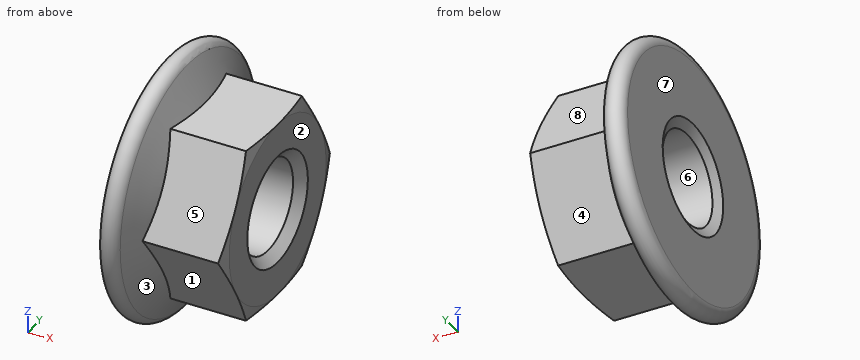
Autodesk Inventor part; units mm, degrees
ref_plane "Work Plane1" through (17.4207, 0, 0) normal (0, 0, -1) x (-1, 0, 0)
ref_plane "YZ Plane" through (0, 0, 0) normal (1, 0, 0) x (0, 1, 0)
ref_plane "XZ Plane" through (0, 0, 0) normal (0, 1, 0) x (-1, 0, 0)
sketch "Sketch1" plane through (0, 0, 0) normal (0, 0, 1) x (1, 0, 0)
  line L0 (-1.1018, 0) -> (6.017, 0)
  line L1 (1.7045, 4) -> (0.9532, 5.6113)
  line L2 (1.7045, 4) -> (5, 4) construction
  line L3 (5, 4) -> (5, 0) construction
  arc A0 (0.9532, 5.6113) -> (0, 5.4) centre (0.5, 5.4) ccw
  line L4 (1.7045, 4) -> (1.7045, 0)
  line L5 (0, -1.1988) -> (0, 7.1926)
  point P0 (0, 0)
  dimension "d2" = 8
  dimension "d4" = 11.8
  dimension "d5" = 0.5
  dimension "d15" = 5
  dimension "d16" = 25
revolve "Ring" add sketch "Sketch1" angle 360 about axis through (-10, 0, 0) along (1, 0, 0)
sketch "Sketch2" plane through (0, 0, 0) normal (-1, 0, 0) x (0, 0, 1)
  circle A0 centre (0, 0) radius 4.9
  line L0 (-4, -2.3094) -> (-4, 2.3094)
  line L1 (-4, 2.3094) -> (0, 4.6188)
  line L2 (0, 4.6188) -> (4, 2.3094)
  line L3 (4, 2.3094) -> (4, -2.3094)
  line L4 (4, -2.3094) -> (0, -4.6188)
  line L5 (0, -4.6188) -> (-4, -2.3094)
  circle A1 centre (0, 0) radius 5.4
  dimension "d6" = 9.2376
extrude "Body" add sketch "Sketch2" against normal blind 5 contours L0 L1 L2 L3 L4 L5
sketch "Sketch3" plane through (0, 0, 0) normal (0, 0, 1) x (1, 0, 0)
  line L0 (1.416, 4.6188) -> (5, 4.6188)
  line L1 (5, 2.3094) -> (5, 4.6188)
  line L2 (0, -5.4) -> (0, 5.4)
  line L3 (-1, 0) -> (6, 0)
  line L4 (4.8342, 4.6188) -> (5, 4)
  dimension "d10" = 15
  dimension "d11" = 8
revolve "Chamfer1" cut sketch "Sketch3" angle 360 about axis through (-10, 0, 0) along (1, 0, 0)
sketch "Sketch4" plane through (0, 0, 0) normal (-1, 0, 0) x (0, 0, 1)
  circle A0 centre (0, 0) radius 5.4
hole "Thread" at (0, 0, 0) direction (1, 0, 0) diameter 4.134 end through all
chamfer "Chamfer2" distance 0.433 angle 30 1 edges at (0, 0, -2.067) measured on face at (0, 4.2317, -0.5138)
ref_plane "Work Plane1" through (17.4207, 0, 0) normal (0, 0, -1) x (-1, 0, 0)
chamfer "Chamfer3" distance 0.433 angle 45 1 edges at (5, 0, -2.067)
equation "\"d6\" = 1.1547 * SW"
equation "\"d7\" = KOH"
equation "\"d12\" = -0.5 * GD1 + 0.5 * NND"
equation "\"d46\" = -0.5 * GD1 + 0.5 * NND"
equation "\"d51\" = -0.5 * GD1 + 0.5 * NND"
equation "\"d2\" = SW"
equation "\"d4\" = LADI"
equation "\"d5\" = PHH"
equation "\"d15\" = KOH"
equation "\"d16\" = KEWI"
equation "\"d10\" = ANG1"
equation "\"d11\" = SW0"
equation "\"ANG1\" = 15deg"
equation "\"KEWI\" = 25deg"
equation "\"NND\" = 5"
equation "\"LADI\" = 11.8"
equation "\"SW\" = 8"
equation "\"PHH\" = RR"
equation "\"KOH\" = 5"
equation "\"SW0\" = SW"
equation "\"d1\" = LADI"
equation "\"d3\" = PHH"
equation "\"GUL\" = 0.541266 * PTC"
equation "\"RR\" = 0.5"
equation "\"THREADDIA\" = 5"
equation "\"TOA\" = 30deg"
equation "\"PTC\" = 0.8"
equation "\"GAL\" = 0.541266 * PTC"
equation "\"E0\" = 1.155 * SW"
properties part number "DIN EN 1661 - M5" material "Steel, Mild"
Read the model definition and answer for the solid it produces. Units are mm, in the model's axes. Face numbers are marked on the shaded views. A direction names the side the tool comes from. Round coordinates to 2 decimals unless told otherwise and drop trailing zeros. Loops run counter-clockwise (first coordinate to the right, second up) from the corner with the lowest first, then second, coordinate; pieces in that order, holes last.
Q1. Consider probe 1 along Z at (x, y) = (2.8, 0); probe 2 along Z at (x, y) = (2.25, 1); probe 3 along Y at (x, z) = (1.15, -1.5). Determine where each line is inside the solid, lowest interval first.
Q2. Section B-B on x = 0.6 is taken. Write down the section's boundary in (y, z).
Q3. Determine the mould class of the marked faces 6, 7 and 8 for opening direction Y: released by +Y, released by -Y, zero draft, split by the parting line, or undercut.
Q4. Which of the six approach directions +Z, -Z, +X, -X, +Y, -Y give full straight-line access (tool end or side, diameter ignored) to the marked faces 1, 2, 3, 4 and 5?
Q5. Each of these flat-tipped pins is pushed along its axis until it touches: pin 1 (1.1 mm diameter, centred on x = 3, y = -0.5, fed in from -Z); pin 2 (2 mm diameter, centred on x = 4, z = 2, fed in from -Y); pin 3 (1.8 mm diameter, centred on x = 3.5, y = -0.5, fed in from +Z). Where does it stop, or does it pass through?
Q6. Section A-A on x = 3.4 is taken. Write down the section's boundary in (y, z), and give its area (3 significant figures).
Output:
1. probe 1: z = -4 to -2.07, 2.07 to 4
1. probe 2: z = -4 to -1.81, 1.81 to 4
1. probe 3: y = -4.97 to -1.42, 1.42 to 4.97
2. outline: circle Ø11.78 at (0, 0); hole circle Ø4.13 at (0, 0)
3. face 6: undercut
3. face 7: zero draft
3. face 8: released by +Y
4. face 1: -Z, +X, -Y
4. face 2: +Z, -Z, +X, +Y, -Y
4. face 3: +X
4. face 4: -Z, +X, +Y
4. face 5: +Z, +X, -Y
5. pin 1: stops at z = -4
5. pin 2: stops at y = -4.04
5. pin 3: stops at z = 4
6. outline: (-4.62, 0) - (-2.31, -4) - (2.31, -4) - (4.62, 0) - (2.31, 4) - (-2.31, 4) - close; hole circle Ø4.13 at (0, 0)
6. area: 42.0 mm2
